Design review of the part built by this model. Coordinates are the model's own, in mm. A direction names the side the tool comes from. Round coordinates to 2 decimals unless told otherwise and drop trailing zeros. Write each loop counter-clockwise with the first axis right and the second up, starting at its lowest first coordinate (ties: lowest second). Pieces come first, ordered by that corner, then holes. Notation, with made-up numbers: M 43,51.5 L 49,51.5 A21 cw 49,58.5 Z; hole C 46.5,36 d3. An arc over 180 degrees is marked long. Use CSV: the item, a comma, the result in double quotes.
from build123d import *

# Parameters (mm, degrees)
SKETCH1_W           = 85
SKETCH1_H           = 190
BOSS_EXTRUDE1_DEPTH = 6
SKETCH2_W           = 73
SKETCH2_H           = 53
CUT_EXTRUDE1_DEPTH  = 4
SKETCH3_R           = 2.1
CUT_EXTRUDE2_DEPTH  = 9
SKETCH4_W           = 25
SKETCH4_H           = 35
CUT_EXTRUDE3_DEPTH  = 10
SKETCH5_W           = 1.5
SKETCH5_H           = 190
CUT_EXTRUDE4_DEPTH  = 10
SKETCH6_W           = 35
SKETCH6_H           = 21.5
CUT_EXTRUDE5_DEPTH  = 2.25
FILLET1_R           = 5


with BuildPart() as part:
    # Sketch1 → Boss-Extrude1 (new body)
    with BuildSketch(Plane(origin=(0, 0, 0), x_dir=(1, 0, 0), z_dir=(0, 1, 0))):
        Rectangle(SKETCH1_W, SKETCH1_H)
    extrude(amount=BOSS_EXTRUDE1_DEPTH)

    # Sketch2 → Cut-Extrude1 (cut)
    with BuildSketch(Plane(origin=(0, 6, 0), x_dir=(1, 0, 0), z_dir=(0, 1, 0))):
        Rectangle(SKETCH2_W, SKETCH2_H)
    extrude(amount=-CUT_EXTRUDE1_DEPTH, mode=Mode.SUBTRACT)

    # Sketch3 → Cut-Extrude2 (cut)
    with BuildSketch(Plane(origin=(0, 6, 0), x_dir=(1, 0, 0), z_dir=(0, 1, 0))):
        with Locations((34, -88)):
            Circle(SKETCH3_R)
        with Locations((-34, -88)):
            Circle(SKETCH3_R)
        with Locations((-34, 88)):
            Circle(SKETCH3_R)
        with Locations((34, 88)):
            Circle(SKETCH3_R)
    extrude(amount=-CUT_EXTRUDE2_DEPTH, mode=Mode.SUBTRACT)

    # Sketch4 → Cut-Extrude3 (cut)
    with BuildSketch(Plane(origin=(0, 6, 0), x_dir=(1, 0, 0), z_dir=(0, 1, 0))):
        with Locations((-30, 59.5)):
            Rectangle(SKETCH4_W, SKETCH4_H)
        with Locations((-30, -59.5)):
            Rectangle(SKETCH4_W, SKETCH4_H)
        with Locations((30, -59.5)):
            Rectangle(SKETCH4_W, SKETCH4_H)
        with Locations((30, 59.5)):
            Rectangle(SKETCH4_W, SKETCH4_H)
    extrude(amount=-CUT_EXTRUDE3_DEPTH, mode=Mode.SUBTRACT)

    # Sketch5 → Cut-Extrude4 (cut)
    with BuildSketch(Plane(origin=(0, 6, 0), x_dir=(1, 0, 0), z_dir=(0, 1, 0))):
        with Locations((-41.75, 0)):
            Rectangle(SKETCH5_W, SKETCH5_H)
        with Locations((41.75, 0)):
            Rectangle(SKETCH5_W, SKETCH5_H)
    extrude(amount=-CUT_EXTRUDE4_DEPTH, mode=Mode.SUBTRACT)

    # Sketch6 → Cut-Extrude5 (cut)
    with BuildSketch(Plane(origin=(0, 6, 0), x_dir=(1, 0, 0), z_dir=(0, 1, 0))):
        with Locations((0, -52.75)):
            Rectangle(SKETCH6_W, SKETCH6_H)
    extrude(amount=-CUT_EXTRUDE5_DEPTH, mode=Mode.SUBTRACT)

    # Fillet1
    fillet1_edges = [part.edges().sort_by_distance(p)[0] for p in [
        (41, 3, -77),
        (-41, 3, 77),
        (-41, 3, -42),
        (-41, 3, 42),
        (-41, 3, -95),
        (-41, 3, -77),
        (-41, 3, 95),
        (41, 3, 42),
        (41, 3, -42),
        (41, 3, 95),
        (41, 3, 77),
        (41, 3, -95),
        (17.5, 3, -42),
        (17.5, 3, -77),
        (-17.5, 1.875, 42),
        (-17.5, 3, 77),
        (17.5, 3, 77),
        (17.5, 1.875, 42),
        (-17.5, 3, -77),
        (-17.5, 3, -42),
    ]]
    fillet(fillet1_edges, radius=FILLET1_R)


solid = part.part
1) Machinability: for faces 4 (the face through (-1, 3, -95)), 5 (the face through (-1, 3, 95)), 6 (the face through (-18.93, 2.96, 75.5)), 7 (the face through (17.5, 2, 60)), 8 (the face through (-1, 4, 26.5)), which of the approach directions +Z, -Z, +X, -X, +Y, -Y give a long, thin tool a straight path to every point of the face, cutting with its end or side? Answer none if there is none.
Answers:
face 4,"-Z, +X, -X, +Y, -Y"
face 5,"+Z, +X, -X, +Y, -Y"
face 6,"-X, +Y, -Y"
face 7,"+X, +Y, -Y"
face 8,"+Y"
2) For pin 1 Ø3 at (y, z) = (2.5, 63.5) entering from -X; pin 2 Ø10 at (x, z) = (27, -49) entering from -Y; pin 3 Ø3 at (y, z) = (4.5, 70.5) entering from +X, all flat-tipped, find the tip position at first contact; note any pin that passes through.
Answers:
pin 1,"x = -17.5"
pin 2,"through"
pin 3,"x = 17.5"
3) Add section B-B on z = 88. Write out the cut boundary in (x, y), then the cut area to 3 significant figures.
Answers:
outline,"M -41,0 L -36.1,0 L -36.1,6 L -41,6 Z; M -31.9,0 L 31.9,0 L 31.9,6 L -31.9,6 Z; M 36.1,0 L 41,0 L 41,6 L 36.1,6 Z"
area,"442 mm²"
4) The part is to be moulded in two halves that separate along Z. For faces 1 (the face through (-41, 3, -86)), 2 (the face through (-19, 2.96, -75.57)), 3 (the face through (-39, 3, 94)), say which applies: released by +Z, released by -Z, zero draft, split by the parting line, or undercut.
Answers:
face 1,"zero draft"
face 2,"undercut"
face 3,"released by +Z"
5) Add section C-C on x = -11. Write out the cut boundary in (y, z), then the cut area to 3 significant figures.
Answers:
outline,"M 0,-95 L 6,-95 L 6,-26.5 L 2,-26.5 L 2,26.5 L 6,26.5 L 6,42 L 3.75,42 L 3.75,63.5 L 6,63.5 L 6,95 L 0,95 Z"
area,"880 mm²"
6) Wall thickness on line 1 along X through (y, z) = (2.9, -88); line 2 along Z through (x, y) = (-24, 0.3); line 3 along Z through (x, y) = (-2, 3.85): over which ranges is each line inside the solid? List them lowest first. Write a range as [from, to].
Answers:
line 1,"[-41, -36.1], [-31.9, 31.9], [36.1, 41]"
line 2,"[-95, -77], [-42, 42], [77, 95]"
line 3,"[-95, -26.5], [26.5, 42], [63.5, 95]"
7) Add section A-A on x = -34. Write out the cut boundary in (y, z), then the cut area to 3 significant figures.
Answers:
outline,"M 0,-95 L 6,-95 L 6,-90.1 L 0,-90.1 Z; M 0,-85.9 L 6,-85.9 L 6,-77 L 0,-77 Z; M 0,-42 L 6,-42 L 6,-26.5 L 2,-26.5 L 2,26.5 L 6,26.5 L 6,42 L 0,42 Z; M 0,77 L 6,77 L 6,85.9 L 0,85.9 Z; M 0,90.1 L 6,90.1 L 6,95 L 0,95 Z"
area,"458 mm²"
